from build123d import *

# Parameters (mm, degrees)
SKETCH1_R           = 1.599999999999998
SKETCH1_R_2         = 1.5999999999996972
SKETCH1_R_3         = 1.6000000000003676
SKETCH1_R_4         = 1.600000000000762
SKETCH1_R_5         = 1.6000000000001544
SKETCH1_R_6         = 1.5999999999994483
BOSS_EXTRUDE1_DEPTH = 7.5
BOSS_EXTRUDE2_START = -15
BOSS_EXTRUDE2_DEPTH = 15
SKETCH3_R           = 1.5999999999999979
CUT_EXTRUDE1_DEPTH  = 15
FILLET3_R           = 2
FILLET4_R           = 2
FILLET5_R           = 2
FILLET6_R           = 2


with BuildPart() as part:
    # Sketch1 → Boss-Extrude1 (new body)
    with BuildSketch(Plane(origin=(0, 0, 0), x_dir=(1, 0, 0), z_dir=(0, 1, 0))):
        with BuildLine():
            Line((-5.000000000000007, 43.96660664640836), (-5.000000000000007, 44.52010781658104))
            ThreePointArc((-5.000000000000007, 44.52010781658104), (-7.2e-15, 44.8), (4.999999999999993, 44.52010781658104))
            Line((4.999999999999993, 44.52010781658104), (4.999999999999993, 43.966606646408366))
            ThreePointArc((4.999999999999993, 43.966606646408366), (31.289475067504778, 31.289475067504675), (43.96660664640838, 4.9999999999998535))
            Line((43.96660664640838, 4.9999999999998535), (44.52010781658105, 4.999999999999852))
            ThreePointArc((44.52010781658105, 4.999999999999852), (44.8, -1.4984e-13), (44.52010781658102, -5.000000000000148))
            Line((44.52010781658102, -5.000000000000148), (43.966606646408344, -5.0000000000001465))
            ThreePointArc((43.966606646408344, -5.0000000000001465), (31.289475067504558, -31.289475067504878), (4.9999999999997, -43.96660664640838))
            Line((4.9999999999997, -43.96660664640838), (4.999999999999696, -44.52010781658105))
            ThreePointArc((4.999999999999696, -44.52010781658105), (-3.0563e-13, -44.79999999999998), (-5.000000000000304, -44.52010781658099))
            Line((-5.000000000000304, -44.52010781658099), (-5.0000000000003, -43.966606646408316))
            ThreePointArc((-5.0000000000003, -43.966606646408316), (-31.289475067505, -31.28947506750445), (-43.96660664640841, -4.999999999999546))
            Line((-43.96660664640841, -4.999999999999546), (-44.52010781658109, -4.999999999999541))
            ThreePointArc((-44.52010781658109, -4.999999999999541), (-44.8, 4.6308e-13), (-44.52010781658098, 5.00000000000046))
            Line((-44.52010781658098, 5.00000000000046), (-43.96660664640831, 5.000000000000454))
            ThreePointArc((-43.96660664640831, 5.000000000000454), (-31.289475067504558, 31.289475067504895), (-5.000000000000007, 43.96660664640836))
        make_face()
        with Locations(Location((36.25, 0, 0), (0, 0, 270))):
            Circle(SKETCH1_R, mode=Mode.SUBTRACT)
        with Locations(Location((8.9734e-13, -36.25, 0), (0, 0, 270))):
            Circle(SKETCH1_R_2, mode=Mode.SUBTRACT)
        with Locations(Location((-25.63262081801145, -25.63262081801235, 0), (0, 0, 270))):
            Circle(SKETCH1_R_3, mode=Mode.SUBTRACT)
        with Locations(Location((-36.249999999999105, -4.44e-15, 0), (0, 0, 270))):
            Circle(SKETCH1_R_4, mode=Mode.SUBTRACT)
        with Locations(Location((8.8846e-13, 36.25, 0), (0, 0, 270))):
            Circle(SKETCH1_R_5, mode=Mode.SUBTRACT)
        with Locations(Location((25.632620818013237, 25.632620818012352, 0), (0, 0, 270))):
            Circle(SKETCH1_R_6, mode=Mode.SUBTRACT)
        with BuildLine():
            Line((33.43022604609433, 5), (36.58637041303769, 5))
            ThreePointArc((36.58637041303769, 5), (38.12774607334069, 5.725574218000316), (38.55073929427462, 7.375838926174497))
            ThreePointArc((38.55073929427462, 7.375838926174497), (36.262271651068, 15.02032472032978), (32.474994896373964, 22.0439834530986))
            ThreePointArc((32.474994896373964, 22.0439834530986), (31.00898015555284, 22.911795444083076), (29.406004523994554, 22.33493671212909))
            Line((29.406004523994554, 22.33493671212909), (27.174273439725177, 20.10320562785971))
            ThreePointArc((27.174273439725177, 20.10320562785971), (25.76005987735207, 19.517419190232797), (24.345846314978967, 20.10320562785971))
            Line((24.345846314978967, 20.10320562785971), (20.1032056278597, 24.345846314978974))
            ThreePointArc((20.1032056278597, 24.345846314978974), (19.51741919023278, 25.76005987735208), (20.103205627859698, 27.174273439725187))
            Line((20.103205627859698, 27.174273439725187), (22.33493671212907, 29.406004523994557))
            ThreePointArc((22.33493671212907, 29.406004523994557), (22.91179544408306, 31.00898015555285), (22.043983453098583, 32.474994896373985))
            ThreePointArc((22.043983453098583, 32.474994896373985), (15.02032472032976, 36.26227165106802), (7.37583892617449, 38.55073929427462))
            ThreePointArc((7.37583892617449, 38.55073929427462), (5.725574218000309, 38.12774607334069), (4.999999999999993, 36.58637041303769))
            Line((4.999999999999993, 36.58637041303769), (4.999999999999994, 33.43022604609433))
            ThreePointArc((4.999999999999994, 33.43022604609433), (4.4142135623730905, 32.01601248372122), (2.9999999999999796, 31.430226046094315))
            Line((2.9999999999999796, 31.430226046094315), (-2.999999999999992, 31.430226046094315))
            ThreePointArc((-2.999999999999992, 31.430226046094315), (-4.414213562373101, 32.01601248372123), (-5.000000000000006, 33.43022604609433))
            Line((-5.000000000000006, 33.43022604609433), (-5.000000000000007, 36.58637041303769))
            ThreePointArc((-5.000000000000007, 36.58637041303769), (-5.7255742180003235, 38.12774607334069), (-7.375838926174504, 38.55073929427462))
            ThreePointArc((-7.375838926174504, 38.55073929427462), (-27.753941161571994, 27.753941161571998), (-38.55073929427462, 7.3758389261744925))
            ThreePointArc((-38.55073929427462, 7.3758389261744925), (-38.12774607334069, 5.725574218000312), (-36.58637041303769, 4.999999999999996))
            Line((-36.58637041303769, 4.999999999999996), (-33.43022604609433, 4.9999999999999964))
            ThreePointArc((-33.43022604609433, 4.9999999999999964), (-32.01601248372122, 4.414213562373094), (-31.430226046094315, 2.9999999999999822))
            Line((-31.430226046094315, 2.9999999999999822), (-31.430226046094315, -2.9999999999999893))
            ThreePointArc((-31.430226046094315, -2.9999999999999893), (-32.01601248372123, -4.4142135623730985), (-33.43022604609433, -5.0000000000000036))
            Line((-33.43022604609433, -5.0000000000000036), (-36.58637041303769, -5.000000000000004))
            ThreePointArc((-36.58637041303769, -5.000000000000004), (-38.12774607334069, -5.725574218000321), (-38.55073929427462, -7.375838926174501))
            ThreePointArc((-38.55073929427462, -7.375838926174501), (-36.26227165106801, -15.02032472032978), (-32.47499489637397, -22.043983453098594))
            ThreePointArc((-32.47499489637397, -22.043983453098594), (-31.008980155552848, -22.911795444083076), (-29.406004523994554, -22.334936712129085))
            Line((-29.406004523994554, -22.334936712129085), (-27.17427343972518, -20.103205627859708))
            ThreePointArc((-27.17427343972518, -20.103205627859708), (-25.760059877352074, -19.517419190232793), (-24.34584631497897, -20.103205627859708))
            Line((-24.34584631497897, -20.103205627859708), (-20.103205627859705, -24.34584631497897))
            ThreePointArc((-20.103205627859705, -24.34584631497897), (-19.517419190232783, -25.760059877352074), (-20.1032056278597, -27.174273439725184))
            Line((-20.1032056278597, -27.174273439725184), (-22.334936712129075, -29.406004523994554))
            ThreePointArc((-22.334936712129075, -29.406004523994554), (-22.911795444083065, -31.008980155552848), (-22.043983453098587, -32.47499489637398))
            ThreePointArc((-22.043983453098587, -32.47499489637398), (-15.020324720329771, -36.262271651068005), (-7.375838926174493, -38.55073929427462))
            ThreePointArc((-7.375838926174493, -38.55073929427462), (-5.725574218000314, -38.12774607334069), (-4.999999999999997, -36.58637041303769))
            Line((-4.999999999999997, -36.58637041303769), (-4.999999999999998, -33.43022604609433))
            ThreePointArc((-4.999999999999998, -33.43022604609433), (-4.414213562373095, -32.01601248372122), (-2.999999999999984, -31.430226046094315))
            Line((-2.999999999999984, -31.430226046094315), (2.9999999999999876, -31.430226046094315))
            ThreePointArc((2.9999999999999876, -31.430226046094315), (4.414213562373097, -32.01601248372123), (5.000000000000002, -33.43022604609433))
            Line((5.000000000000002, -33.43022604609433), (5.000000000000003, -36.58637041303769))
            ThreePointArc((5.000000000000003, -36.58637041303769), (5.725574218000319, -38.12774607334069), (7.3758389261745, -38.55073929427462))
            ThreePointArc((7.3758389261745, -38.55073929427462), (27.753941161571998, -27.753941161571994), (38.55073929427462, -7.375838926174497))
            ThreePointArc((38.55073929427462, -7.375838926174497), (38.12774607334069, -5.725574218000316), (36.58637041303769, -5))
            Line((36.58637041303769, -5), (33.43022604609433, -5))
            ThreePointArc((33.43022604609433, -5), (32.01601248372123, -4.414213562373095), (31.430226046094315, -2.999999999999986))
            Line((31.430226046094315, -2.999999999999986), (31.430226046094315, 2.999999999999986))
            ThreePointArc((31.430226046094315, 2.999999999999986), (32.01601248372123, 4.414213562373095), (33.43022604609433, 5))
        make_face(mode=Mode.SUBTRACT)
    extrude(amount=BOSS_EXTRUDE1_DEPTH)

    # Sketch2 → Boss-Extrude2 (add)
    with BuildSketch(Plane(origin=(0, 7.5, 0), x_dir=(1, 0, 0), z_dir=(0, 1, 0)).offset(BOSS_EXTRUDE2_START)):
        with BuildLine():
            Line((-30.348716864560213, 32.202762065927786), (-22.924095662101468, 24.778140863469048))
            ThreePointArc((-22.924095662101468, 24.778140863469048), (-21.509882099728365, 24.192354425842133), (-20.095668537355262, 24.778140863469048))
            Line((-20.095668537355262, 24.778140863469048), (-17.620794803202365, 27.253014597621945))
            ThreePointArc((-17.620794803202365, 27.253014597621945), (-17.03500836557545, 28.66722815999505), (-17.620794803202365, 30.081441722368155))
            Line((-17.620794803202365, 30.081441722368155), (-24.43259094183973, 36.89323786100552))
            ThreePointArc((-24.43259094183973, 36.89323786100552), (-27.490872340486693, 34.674406093818874), (-30.348716864560213, 32.202762065927786))
        make_face()
        with BuildLine():
            Line((24.778140863469044, -20.09566853735524), (27.253014597621938, -17.620794803202347))
            ThreePointArc((27.253014597621938, -17.620794803202347), (28.66722815999504, -17.035008365575433), (30.081441722368144, -17.620794803202347))
            Line((30.081441722368144, -17.620794803202347), (36.89323786100551, -24.4325909418397))
            ThreePointArc((36.89323786100551, -24.4325909418397), (34.67440609381886, -27.49087234048667), (32.20276206592778, -30.348716864560195))
            Line((32.20276206592778, -30.348716864560195), (24.778140863469044, -22.924095662101447))
            ThreePointArc((24.778140863469044, -22.924095662101447), (24.19235442584213, -21.509882099728344), (24.778140863469044, -20.09566853735524))
        make_face()
    extrude(amount=BOSS_EXTRUDE2_DEPTH)

    # Sketch3 → Cut-Extrude1 (cut)
    with BuildSketch(Plane(origin=(0.9270226006838173, 0, -0.9270226006838158), x_dir=(0.7071067811865471, 0, 0.7071067811865479), z_dir=(-0.7071067811865479, 0, 0.7071067811865471))):
        with Locations((-38, -4.5)):
            Circle(SKETCH3_R)
        with Locations(Location((38, -4.49999999999999, 0), (0, 0, 180))):
            Circle(SKETCH3_R)
    extrude(amount=-CUT_EXTRUDE1_DEPTH, mode=Mode.SUBTRACT)

    # Fillet3
    fillet3_edges = [part.edges().sort_by_distance(p)[0] for p in [
        (28.665477480107445, 3.75, 26.811432278739854),
        (30.434119773017613, 0, 28.58007457165003),
    ]]
    fillet(fillet3_edges, radius=FILLET3_R)

    # Fillet4
    fillet4_edges = [part.edges().sort_by_distance(p)[0] for p in [
        (33.27592050584852, 3.75, 20.815273586682707),
        (35.08457918342702, 8.9e-16, 22.623932264261207),
    ]]
    fillet(fillet4_edges, radius=FILLET4_R)

    # Fillet5
    fillet5_edges = [part.edges().sort_by_distance(p)[0] for p in [
        (-20.815273586682718, 3.75, -33.275920505848504),
        (-22.62393226426122, 0, -35.08457918342701),
    ]]
    fillet(fillet5_edges, radius=FILLET5_R)

    # Fillet6
    fillet6_edges = [part.edges().sort_by_distance(p)[0] for p in [
        (-26.811432278739865, 3.75, -28.66547748010744),
        (-28.580074571650037, 8.9e-16, -30.434119773017613),
    ]]
    fillet(fillet6_edges, radius=FILLET6_R)


solid = part.part
Verification items for the finished model (mm, model axes). A direction names the side the tool comes from. Give positions to 0.01 mm unless a question says otherwise; leave off trailing zeros. Order: outer loops, then holes, each group sorted by start corner. A loop starts at its lowest first (then second) coordinate and runs counter-clockwise, first axis right, second up. Notation, with made-up numbers: M -27,-12.75 L 29,-12.75 A16 ccw 29,11.25 Z; hole C 18,40.25 d10. An arc over 180 degrees is marked long. Use one line per item in the form item = value. Start each with the question number.
Q1. Access from +Z, -Z, +X, -X, +Y, -Y to the whole of each face (thin tool, end or side, straight path). Record for faces 4 (the flat face through (-19.47, -3.44, -31.93)), 5 (the cylindrical face through (-0.1, 3.7, -44.8)), 6 (the cylindrical face through (28.645, -0.105, 17.035)).
Q2. Scan lines: line 1 along Z through (x, y) = (21.5, 3); line 2 along X through (y, z) = (5.25, -27); line 3 along X through (y, z) = (5, -36.25). Record each from-to range of solid material in increasing order. Write a range as [from, to].
Q3. Mould release check, pull along Z, two halves, no side actions. Record for faces 1 (the cylindrical face through (-38.112, 3.698, 5.707)), 2 (the flat face through (31, -7.5, 24)), 3 (the cylindrical face through (31.583, 3.228, 30.994)): +Z half, -Z half, draft (parallel to the pull), parting line (faces both ways), or undercut.
Q4. Section check D-D (y = 1.75). Count the separate pieces of the cut face and the enclosed holes in it, then the cut area to 3 significant figures.
Q5. Section check B-B (x = -13). Enter the section's corners in (y, z), then the cut area to 3 significant figures.
Q6. Section check C-C (z = 16). Enter the section's corners in (x, y), then the cut area to 3 significant figures.
Q7. Section check A-A (x = 0). Enter the section's corners in (y, z), then the cut area to 3 significant figures.
Q8. Go/stop test with flat-tipped pins: pin 1 Ø2.5 at (x, z) = (-25.63, 25.63) entering from +Y; pin 2 Ø3.5 at (x, y) = (35, 3) entering from -Z; pin 3 Ø3.5 at (x, z) = (-36.25, 0) entering from -Y; pin 4 Ø1.6 at (y, z) = (4.5, -35.5) entering from +X. Record where each tip stops, or that it passes through.
Evaluation:
q1.face_4 = -Y
q1.face_5 = -Z, +Y, -Y
q1.face_6 = +Y, -Y
q2.line_1 = [-38.68, -32.84], [-28.57, -22.95], [32.84, 38.68]
q2.line_2 = [-35.06, -28.49], [-25.15, -17.87], [19.95, 24.8], [26.46, 35.06]
q2.line_3 = [-25.38, -15.05], [-5, -1.6], [1.6, 5], [15.05, 25.38]
q3.face_1 = undercut
q3.face_2 = draft
q3.face_3 = +Z half
q4.separate_pieces = 1
q4.enclosed_holes = 7
q4.area = 1,860 mm2
q5.outline = M 0,-42.3 L 7.5,-42.3 L 7.5,-37.03 L 0,-37.03 Z; M 0,37.03 L 7.5,37.03 L 7.5,42.3 L 0,42.3 Z
q5.area = 78.9 mm2
q6.outline = M -41.26,0 L -35.84,0 L -35.84,7.5 L -41.26,7.5 Z; M 35.84,0 L 41.26,0 L 41.26,7.5 L 35.84,7.5 Z
q6.area = 81.2 mm2
q7.outline = M 0,-44.8 L 7.5,-44.8 L 7.5,-37.85 L 0,-37.85 Z; M 0,-34.65 L 7.5,-34.65 L 7.5,-31.43 L 0,-31.43 Z; M 0,31.43 L 7.5,31.43 L 7.5,34.65 L 0,34.65 Z; M 0,37.85 L 7.5,37.85 L 7.5,44.8 L 0,44.8 Z
q7.area = 153 mm2
q8.pin_1 = through
q8.pin_2 = -29.2
q8.pin_3 = 0
q8.pin_4 = 27.46
